Input: part model. Units: mm. Frame: model coordinates. A direction names the side the tool comes from. Round coordinates to 2 decimals unless told otherwise and drop trailing zeros. Order: outer loops, then holes, each group sorted by start corner. A loop starts at its lowest first (then second) coordinate and runs counter-clockwise, first axis right, second up.
Item 1: Cut plane B-B on z = 70. Output: boundary loops of the cut face in (x, y) (3 decimals), then the cut area to 3 significant figures.
Item 2: First-contact query: pin 1 (5 mm diameter, centred on x = -7, z = 74.5, fed in from +Y); pin 2 (14.5 mm diameter, centred on x = 0, z = 38.1, fed in from +Y) (3 decimals); pin 3 (10 mm diameter, centred on y = 20, z = 36.5, fed in from +X); pin 4 (1 mm diameter, centred on x = -14.5, y = 19, fed in from -Z). Flat tips, straight axial feed; report the tip coordinate or a pass-through.
Item 3: Cut plane A-A on x = 0. Give the number of separate pieces and of enclosed holes in the cut face, then the cut area to 3 significant figures.
Item 4: Line query: L1, parallel to Y at x = 0, z = 47.5 (3 decimals); L2, parallel to Z at x = 0, y = -27.25; L3, parallel to X at y = -27.25, z = 38.1. Output: solid intervals per line, ascending.
Item 5: Mould query, pull axis Z, two halves, no side actions, for faces 3 (the flat face through (2, -26, 144.272)), 4 (the cylindrical face through (0.246, -29.78, 32.517)), 5 (the cylindrical face through (-27.715, -21.251, 133.328)). Classes: released by +Z, released by -Z, zero draft, split by the parting line, or undercut.
Item 6: Cut plane C-C on z = 38.1. Output: boundary loops of the cut face in (x, y) (3 decimals), then the cut area to 3 significant figures.
Item 7: Reachability of faces 1 (the cylindrical face through (-27.715, -21.251, 62.611)), 2 (the cylindrical face through (30.647, 9.651, 129.348)) from +Z, -Z, +X, -X, +Y, -Y: full face, straight path, thin tool, end or side. Return the list, or none.
```python
from build123d import *

# Parameters (mm, degrees)
SKETCH1_R               = 34.925
SKETCH1_R_2             = 25.4
BOSS_EXTRUDE1_DEPTH     = 144.272
CUT_EXTRUDE1_REACH      = 154.492
CUT_EXTRUDE1_END_RADIUS = 34.925
SKETCH2_R               = 5.588


with BuildPart() as part:
    # Sketch1 → Boss-Extrude1 (new body)
    with BuildSketch(Plane.XY):
        Circle(SKETCH1_R)
        Circle(SKETCH1_R_2, mode=Mode.SUBTRACT)
    extrude(amount=BOSS_EXTRUDE1_DEPTH)

    # Cut-Extrude1: up to this cylinder (the profile starts inside it)
    cut_extrude1_end = Plane(origin=(0, 0, 38.1), z_dir=(0, 0, -1)) * Cylinder(CUT_EXTRUDE1_END_RADIUS, 379.834, mode=Mode.PRIVATE)
    # Sketch2 → Cut-Extrude1 (cut, up to the surface)
    with BuildSketch(Plane(origin=(0, 0, 0), x_dir=(1, 0, 0), z_dir=(0, 1, 0)), mode=Mode.PRIVATE) as cut_extrude1_sk1:
        with Locations(Location((0, -38.1, 0), (0, 0, 270))):
            Circle(SKETCH2_R)
    cut_extrude1_tool1 = extrude(cut_extrude1_sk1.sketch, amount=-CUT_EXTRUDE1_REACH, mode=Mode.PRIVATE) & cut_extrude1_end
    add(cut_extrude1_tool1.solids().sort_by_distance((0, 0, 38.1))[0], mode=Mode.SUBTRACT)

    # Cut-Sweep1: sweep along a path in groove path
    with BuildLine(Plane.XY.offset(131.7625)) as cut_sweep1_path:
        CenterArc((0, 0), 34.925, 0, 360)
    # groove → Cut-Sweep1 (sweep, cut)
    with BuildSketch(Plane(origin=(0, 0, 0), x_dir=(0, 0, -1), z_dir=(1, 0, 0))):
        Polygon((-139.7, 34.925), (-139.7, 32.131), (-134.9375, 32.131), (-134.9375, 34.925), (-131.7625, 34.925), (-131.7625, 32.131), (-127, 32.131), (-127, 34.925), (-127, 38.1), (-139.7, 38.1), align=None)
    sweep(path=cut_sweep1_path.line, mode=Mode.SUBTRACT)


solid = part.part
```
From the geometry:
1. outline: circle Ø69.85 at (0, 0); hole circle Ø50.8 at (0, 0)
1. area: 1,810 mm2
2. pin 1: stops at y = 34.63
2. pin 2: stops at y = 34.925
2. pin 3: stops at x = 31.54
2. pin 4: passes through
3. separate pieces: 3
3. enclosed holes: 0
3. area: 2,590 mm2
4. L1: y = -34.925 to -25.4, 25.4 to 34.925
4. L2: z = 0 to 32.51, 43.69 to 144.27
4. L3: x = -21.84 to -5.59, 5.59 to 21.84
5. face 3: released by +Z
5. face 4: undercut
5. face 5: zero draft
6. outline: (-5.588, -34.475) - (-5.588, -24.778) arc R25.4 cw (long way) to (5.588, -24.778) - (5.588, -34.475) arc R34.925 ccw (long way) to start
6. area: 1,700 mm2
7. face 1: +Z, -Z
7. face 2: none
